Here's how the part is built. I have some questions about the finished solid (model axes, mm). Round coordinates to 2 decimals unless told otherwise and drop trailing zeros. Order: outer loops, then holes, each group sorted by start corner. A loop starts at its lowest first (then second) coordinate and runs counter-clockwise, first axis right, second up. Notation, with made-up numbers: M -17.5,38.5 L 22.5,38.5 A28 ccw 22.5,63.5 Z; hole C 87.25,19.5 d10. An arc over 180 degrees is marked long. Answer as CSV lines item,"result". Start each with the question number.
```python
from build123d import *

# Parameters (mm, degrees)
F0_R     = 39
F0_R_2   = 35
F1_DEPTH = 4
F2_R     = 1.99999
F3_R     = 1.99999


# Not quite as in the source:
# - a fillet or chamfer is up to 0.001 mm smaller than in the source, because OpenCascade refuses the exact size


with BuildPart() as f1:
    # F0 (on Top) → F1 (new body)
    with BuildSketch(Plane.XY):
        Circle(F0_R)
        Circle(F0_R_2, mode=Mode.SUBTRACT)
    extrude(amount=F1_DEPTH)

    # F2 (radius 2 in the source; OpenCascade refuses exactly that, so slightly less here)
    f2_edges = [f1.edges().sort_by_distance(p)[0] for p in [
        (-39, 0, 0),
        (-35, 0, 0),
    ]]
    fillet(f2_edges, radius=F2_R)

    # F3 (radius 2 in the source; OpenCascade refuses exactly that, so slightly less here)
    f3_edges = [f1.edges().sort_by_distance(p)[0] for p in [
        (-39, 0, 4),
        (-35, 0, 4),
    ]]
    fillet(f3_edges, radius=F3_R)


solid = f1.part
```
Item 1: For P1, Ø1.5, axis at x = 19.5, z = 3, coming from the +Y side; P2, Ø5, axis at x = 24, y = -23, coming from the +Z side, each with a flat end and sliding along its axis, tell me the tip position at first contact or that it passes through.
Item 2: If I drill on line 1 along Y through (x, z) = (0, 2.05); line 2 along X through (y, z) = (26.5, 1.4); line 3 along Y through (x, z) = (-26, 3.35), over which ranges is the centre line in solid material (lowest first)?
Item 3: If we section it at C-C on z = 0.9: Please give me the cut outline in (x, y).
Geometry says:
1,P1,"y = 34.03"
1,P2,"z = 3.55"
2,line 1,"-39 to -35, 35 to 39"
2,line 2,"-28.49 to -23, 23 to 28.49"
2,line 3,"-28.36 to -24.21, 24.21 to 28.36"
3,outline,"C 0,0 d77.34; hole C 0,0 d70.66"
